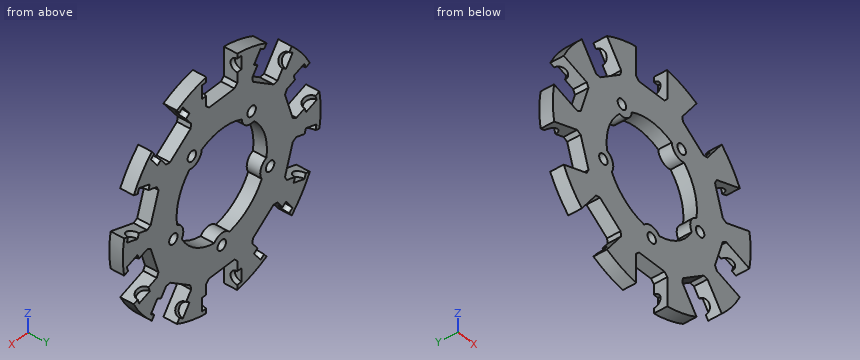
```python
from build123d import *

# Parameters (mm, degrees)
SKIZZE1_R                       = 35
AUFSATZ_LINEAR_AUSTRAGEN1_DEPTH = 4
SCHNITT_LINEAR_AUSTRAGEN1_DEPTH = 5
SKIZZE4_W                       = 14
SKIZZE4_H                       = 2
KREISMUSTER1_COUNT              = 10
SKIZZE5_R                       = 16
SCHNITT_LINEAR_AUSTRAGEN2_DEPTH = 5
SKIZZE7_R                       = 3.5
AUFSATZ_LINEAR_AUSTRAGEN2_DEPTH = 4
SKIZZE6_R                       = 1.5
SCHNITT_LINEAR_AUSTRAGEN3_DEPTH = 5
KREISMUSTER2_COUNT              = 5


with BuildPart() as part:
    # Skizze1 → Aufsatz-Linear austragen1 (new body)
    with BuildSketch(Plane(origin=(0, 0, 0), x_dir=(1, 0, 0), z_dir=(0, 1, 0))):
        Circle(SKIZZE1_R)
    extrude(amount=AUFSATZ_LINEAR_AUSTRAGEN1_DEPTH)

    # Skizze2 → Schnitt-Linear austragen1 (cut, through all)
    with BuildSketch(Plane(origin=(0, 4, 0), x_dir=(1, 0, 0), z_dir=(0, 1, 0))):
        Polygon((-5.5, 37), (-5.5, 26), (-4.5, 25), (0, 25), (4.5, 25), (5.5, 26), (5.5, 37), align=None)
    schnitt_linear_austragen1 = extrude(amount=-SCHNITT_LINEAR_AUSTRAGEN1_DEPTH, mode=Mode.SUBTRACT)

    # Skizze4 → Schnitt-Rotation1 (revolve, cut)
    with BuildSketch(Plane(origin=(0, 4, 0), x_dir=(1, 0, 0), z_dir=(0, 1, 0))):
        with Locations((0, 30.065155865)):
            Rectangle(SKIZZE4_W, SKIZZE4_H)
    schnitt_rotation1 = revolve(axis=Axis((-7, 4, -31.065155865), (1, 0, 0)), mode=Mode.SUBTRACT)

    # Kreismuster1: Schnitt-Linear austragen1, Schnitt-Rotation1 ×10 about axis
    kreismuster1_axis = Axis((0, 0, 0), (0, 1, 0))
    for i in range(1, KREISMUSTER1_COUNT):
        add(schnitt_linear_austragen1.rotate(kreismuster1_axis, i * 360 / KREISMUSTER1_COUNT), mode=Mode.SUBTRACT)
        add(schnitt_rotation1.rotate(kreismuster1_axis, i * 360 / KREISMUSTER1_COUNT), mode=Mode.SUBTRACT)

    # Skizze5 → Schnitt-Linear austragen2 (cut, through all)
    with BuildSketch(Plane(origin=(0, 4, 0), x_dir=(1, 0, 0), z_dir=(0, 1, 0))):
        Circle(SKIZZE5_R)
    extrude(amount=-SCHNITT_LINEAR_AUSTRAGEN2_DEPTH, mode=Mode.SUBTRACT)

    # Skizze7 → Aufsatz-Linear austragen2 (add)
    with BuildSketch(Plane(origin=(0, 0, 0), x_dir=(-1, 0, 0), z_dir=(0, -1, 0))):
        with Locations((0, 18)):
            Circle(SKIZZE7_R)
    aufsatz_linear_austragen2 = extrude(amount=-AUFSATZ_LINEAR_AUSTRAGEN2_DEPTH)

    # Skizze6 → Schnitt-Linear austragen3 (cut, through all)
    with BuildSketch(Plane.XZ):
        with Locations((0, -18)):
            Circle(SKIZZE6_R)
    schnitt_linear_austragen3 = extrude(amount=-SCHNITT_LINEAR_AUSTRAGEN3_DEPTH, mode=Mode.SUBTRACT)

    # Kreismuster2: Aufsatz-Linear austragen2, Schnitt-Linear austragen3 ×5 about axis
    kreismuster2_axis = Axis((0, 0, 0), (0, 1, 0))
    for i in range(1, KREISMUSTER2_COUNT):
        add(aufsatz_linear_austragen2.rotate(kreismuster2_axis, i * 360 / KREISMUSTER2_COUNT))
        add(schnitt_linear_austragen3.rotate(kreismuster2_axis, i * 360 / KREISMUSTER2_COUNT), mode=Mode.SUBTRACT)


solid = part.part
```
Design review of the part built by this model. Coordinates are the model's own, in mm. Give positions to 0.01 mm unless a question says otherwise; leave off trailing zeros. Order: outer loops, then holes, each group sorted by start corner. A loop starts at its lowest first (then second) coordinate and runs counter-clockwise, first axis right, second up. Notation, with made-up numbers: (13, 25) - (32, 25) arc R32 ccw to (32, 61) - close; hole circle Ø5 at (-4, 25). An arc over 180 degrees is marked (long way). Use a Markdown table: item, result. Add a question column.
(1) Add section B-B on x = 0. Give the boundary of the cut face in (y, z), then the cut area to 3 significant figures.
(2) Clearance check with flat-ended pins moving along their axes: P1, Ø2, axis at x = 1.5, y = 1.5, coming from the +Z side; P2, Ø0.6, axis at y = 3, z = -30.5, coming from the +X side; P3, Ø2.5, axis at x = 0, z = -18, coming from the -Y side (1 decimal); P4, Ø1.2, axis at y = 1.5, z = -30.5, coming from the -X side. State where each tip first meets the part, or that it passes through.
(3) Wall thickness on probe 1 along X at (y, z) = (0.8, -10.5); probe 2 along X at (y, z) = (2.45, -30); probe 3 along Z at (x, y) = (0, 2.6): over which ranges is each line inside the solid? List them lowest first. Write a range as [from, to].
(4) Add section A-A on z = -0.5. Give the boundary of the cut face in (x, y), then the cut area to 3 significant figures.
Report:
| question | item | result |
|---|---|---|
| 1 | outline | (0, -25) - (4, -25) - (4, -19.5) - (0, -19.5) - close; (0, -16.5) - (4, -16.5) - (4, -14.5) - (0, -14.5) - close; (0, 16) - (4, 16) - (4, 25) - (0, 25) - close |
| 1 | area | 66.0 mm² |
| 2 | P1 | stops at z = 25 |
| 2 | P2 | stops at x = 15.58 |
| 2 | P3 | passes through |
| 2 | P4 | stops at x = -15.8 |
| 3 | probe 1 | x = [-22.87, -12.07], [12.07, 22.87] |
| 3 | probe 2 | x = [-15, -13.71], [-13.14, -7], [7, 13.14], [13.71, 15] |
| 3 | probe 3 | z = [-25, -19.5], [-16.5, -14.5], [16, 25] |
| 4 | outline | (-35, 0) - (-15.99, 0) - (-15.99, 4) - (-35, 4) - close; (15.99, 0) - (35, 0) - (35, 4) - (15.99, 4) - close |
| 4 | area | 152 mm² |
